```python
from build123d import *

# Parameters (mm, degrees)
SKETCH1_W           = 100
SKETCH1_H           = 12.7
SKETCH1_R           = 1.75
BOSS_EXTRUDE1_DEPTH = 12
SKETCH2_R           = 3
CUT_EXTRUDE1_DEPTH  = 3.5
SKETCH3_R           = 1.6
CUT_EXTRUDE2_DEPTH  = 50
SKETCH4_R           = 2
CUT_EXTRUDE3_DEPTH  = 7
FILLET1_R           = 2
FILLET2_R           = 1.5
BOSS_EXTRUDE2_START = 0.8
SKETCH5_W           = 7.5
SKETCH5_H           = 7.5
SKETCH5_R           = 1.75
BOSS_EXTRUDE2_DEPTH = 0.8
FILLET3_R           = 0.6
FILLET4_R           = 0.5


with BuildPart() as part:
    # Sketch1 → Boss-Extrude1 (new body)
    with BuildSketch(Plane(origin=(0, 0, 0), x_dir=(1, 0, 0), z_dir=(0, 1, 0))):
        with Locations((0, -2.35)):
            Rectangle(SKETCH1_W, SKETCH1_H)
        with Locations(Location((46, 0, 0), (0, 0, 270))):
            Circle(SKETCH1_R, mode=Mode.SUBTRACT)
        with Locations(Location((-46, 0, 0), (0, 0, 90))):
            Circle(SKETCH1_R, mode=Mode.SUBTRACT)
    extrude(amount=BOSS_EXTRUDE1_DEPTH)

    # Sketch2 → Cut-Extrude1 (cut)
    with BuildSketch(Plane(origin=(0, 12, 0), x_dir=(1, 0, 0), z_dir=(0, 1, 0))):
        with Locations(Location((46, 0, 0), (0, 0, 270))):
            Circle(SKETCH2_R)
        with Locations(Location((-46, 0, 0), (0, 0, 270))):
            Circle(SKETCH2_R)
    extrude(amount=-CUT_EXTRUDE1_DEPTH, mode=Mode.SUBTRACT)

    # Sketch3 → Cut-Extrude2 (cut)
    with BuildSketch(Plane.XY.offset(8.7)):
        with Locations((40, 6)):
            Circle(SKETCH3_R)
        with Locations((0, 6)):
            Circle(SKETCH3_R)
        with Locations((-40, 6)):
            Circle(SKETCH3_R)
    extrude(amount=-CUT_EXTRUDE2_DEPTH, mode=Mode.SUBTRACT)

    # Sketch4 → Cut-Extrude3 (cut)
    with BuildSketch(Plane(origin=(0, 0, 8.7), x_dir=(-1, 0, 0), z_dir=(0, 0, -1))):
        with Locations((40, 6)):
            Circle(SKETCH4_R)
        with Locations((0, 6)):
            Circle(SKETCH4_R)
        with Locations((-40, 6)):
            Circle(SKETCH4_R)
    extrude(amount=CUT_EXTRUDE3_DEPTH, mode=Mode.SUBTRACT)

    # Fillet1
    fillet1_edges = [part.edges().sort_by_distance(p)[0] for p in [
        (50, 6, 8.7),
        (-50, 6, 8.7),
    ]]
    fillet(fillet1_edges, radius=FILLET1_R)

    # Fillet2
    # the kernel refuses this fillet: 1.5 mm, written as the material it takes off along each edge
    with BuildSketch(Plane(origin=(-51.75, 12, 8.7), x_dir=(0, -1, 0), z_dir=(1, 0, 0))) as fillet2_piece_1:
        with BuildLine():
            CenterArc((FILLET2_R, FILLET2_R), FILLET2_R, 180, 90)
            Line((0, FILLET2_R), (0, 0))
            Line((0, 0), (FILLET2_R, 0))
        make_face()
    extrude(amount=103.5, mode=Mode.SUBTRACT)

    # Sketch5 → Boss-Extrude2 (add)
    # profile 1 of 2: a face of its own
    with BuildSketch(Plane.XZ.offset(BOSS_EXTRUDE2_START)):
        with Locations((-46, 0)):
            Rectangle(SKETCH5_W, SKETCH5_H)
        with Locations(Location((-46, 0, 0), (0, 0, 270))):
            Circle(SKETCH5_R, mode=Mode.SUBTRACT)
    # profile 2 of 2: a face of its own
    with BuildSketch(Plane.XZ.offset(BOSS_EXTRUDE2_START)):
        with Locations((46, 0)):
            Rectangle(SKETCH5_W, SKETCH5_H)
        with Locations(Location((46, 0, 0), (0, 0, 90))):
            Circle(SKETCH5_R, mode=Mode.SUBTRACT)
    extrude(amount=-BOSS_EXTRUDE2_DEPTH)

    # Fillet3
    fillet3_edges = [part.edges().sort_by_distance(p)[0] for p in [
        (42.25, -0.4, 3.75),
        (42.25, -0.4, -3.75),
        (49.75, -0.4, -3.75),
        (49.75, -0.4, 3.75),
        (-49.75, -0.4, 3.75),
        (-49.75, -0.4, -3.75),
        (-42.25, -0.4, -3.75),
        (-42.25, -0.4, 3.75),
    ]]
    fillet(fillet3_edges, radius=FILLET3_R)

    # Fillet4
    fillet4_edges = [part.edges().sort_by_distance(p)[0] for p in [
        (-50, 12, 1.35),
        (50, 12, 1.35),
        (-49.984059393, 12, 6.952008585),
        (-50, 6, -4),
        (50, 6, -4),
        (49.984059393, 12, 6.952008585),
        (49.135184903, 11.467090552, 8.346619324),
        (-49.135184903, 11.467090552, 8.346619324),
        (0, 12, -4),
    ]]
    fillet(fillet4_edges, radius=FILLET4_R)


solid = part.part
```
Check sheet for the modelled part. Datum: model origin and axes. Units: mm. A direction names the side the tool comes from. Give positions to 0.01 mm unless a question says otherwise; leave off trailing zeros. Loops run counter-clockwise (first coordinate to the right, second up) from the corner with the lowest first, then second, coordinate; pieces in that order, holes last. Notation, with made-up numbers: M 73.25,-36 L 104.25,-36 A13 ccw 104.25,-23 Z; hole C 48.25,65.5 d8. An arc over 180 degrees is marked long. Answer as CSV lines item,"result".
Item 1: Scan lines: L1, parallel to X at y = 11.05, z = 0; L2, parallel to X at y = 4.25, z = 0; L3, parallel to X at y = 5.25, z = 3.25. Record each from-to range of solid material in increasing order.
Reply:
L1,"-50 to -49, -43 to 43, 49 to 50"
L2,"-50 to -47.75, -44.25 to 44.25, 47.75 to 50"
L3,"-50 to -41.85, -38.15 to -1.85, 1.85 to 38.15, 41.85 to 50"
Item 2: Draft check along Y on faces 4 (the face through (-48, 8.5, 0)), 5 (the face through (-1, 0, 2)), 6 (the face through (-49.43, 5.83, 8.1)), 7 (the face through (-0.35, 4.44, -1.11)). Enter one of: pulls with the +Y half, pulls with the -Y half, needs draft (parallel to the pull), parting line crosses it, or undercut.
Reply:
face 4,"pulls with the +Y half"
face 5,"pulls with the -Y half"
face 6,"needs draft"
face 7,"undercut"
Item 3: Sectioned sample at C-C, the plane x = 46. Enter the section's corners in (y, z), then the cut area to 3 significant figures.
Reply:
outline,"M -0.8,-3.75 L 0,-3.75 L 0,-4 L 11.5,-4 A0.5 ccw 12,-3.5 L 12,-3 L 8.5,-3 L 8.5,-1.75 L -0.8,-1.75 Z; M -0.8,1.75 L 8.5,1.75 L 8.5,3 L 12,3 L 12,7.2 A1.5 ccw 10.5,8.7 L 0,8.7 L 0,3.75 L -0.8,3.75 Z"
area,"104 mm^2"
Item 4: Depth check by flat-ended pin: pin 1 Ø5 at (x, z) = (-46, 0) entering from -Y; pin 2 Ø4 at (x, z) = (-46, 0) entering from +Y; pin 3 Ø0.9 at (y, z) = (-0.5, 0) entering from +X; pin 4 Ø6 at (x, z) = (-20, 1) entering from -Y. Enter the tip coordinate at first touch or a pass-through.
Reply:
pin 1,"y = -0.8"
pin 2,"y = 8.5"
pin 3,"x = 49.75"
pin 4,"y = 0"
Item 5: Sectioned sample at A-A, the plane y = 6. State how many separate pieces and enclosed holes the cut face has, then the cut area to 3 significant figures.
Reply:
separate pieces,"4"
enclosed holes,"2"
area,"1,110 mm^2"
Item 6: Set-up check for faces 1 (the face through (49, 10, 0)), 2 (the face through (-40.35, 4.44, -1.11)), 3 (the face through (0, 8, 5)): record each of +Z, -Z, +X, -X, +Y, -Y from which the full face is reachable in a straight line by a thin tool's end or side.
Reply:
face 1,"+Y"
face 2,"+Z, -Z"
face 3,"+Z"
Item 7: Sectioned sample at D-D, the plane y = 1.75. Enter the section's corners in (x, z).
Reply:
outline,"M -50,-3.5 A0.5 ccw -49.5,-4 L 49.5,-4 A0.5 ccw 50,-3.5 L 50,6.7 A2 ccw 48,8.7 L -48,8.7 A2 ccw -50,6.7 Z; hole C -46,0 d3.5; hole C 46,0 d3.5"
